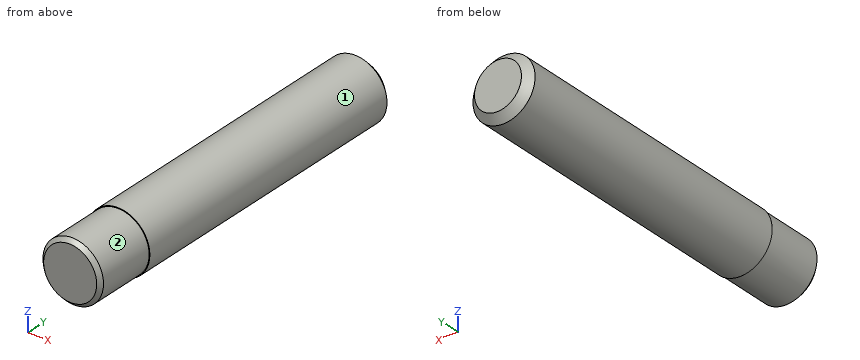
Solid Edge part; units mm, degrees
sketch "Sketch1" plane through (0, 0, 0) normal (0, -1, 0) x (1, 0, 0)
  circle A0 centre (0, 0) radius 4
extrude "Protrusion1" add sketch "Sketch1" along normal mid plane 48
sketch "Sketch2" plane through (0, 24, 0) normal (0, 1, 0) x (1, 0, 0)
  circle A0 centre (0, 0) radius 4.1
extrude "Ausprägung_2" add sketch "Sketch2" against normal blind 40
cosmetic_thread "Thread1"
chamfer "Fase_2" distance 1 angle 45 1 edges at (-4.1, 24, 0)
chamfer "Fase_3" distance 0.5 angle 45 1 edges at (-4, -24, 0)
The model under review builds one solid part; all positions refer to its coordinate system, in mm. Face numbers are marked on the shaded views. A direction names the side the tool comes from. Round coordinates to 2 decimals unless told otherwise and drop trailing zeros. Write each loop counter-clockwise with the first axis right and the second up, starting at its lowest first coordinate (ties: lowest second). Pieces come first, ordered by that corner, then holes. Notation, with made-up numbers: M 86,63 L 145,63 A17 ccw 145,74 Z; hole C 39,-13 d9. An arc over 180 degrees is marked long. Use a Markdown table: item, result. Add a question column.
Q1. Insertion check: pin 1 (2 mm diameter, centred on x = 2.5, y = 16, fed in from +Z); pin 2 (1.5 mm diameter, centred on x = -3, y = 18, fed in from +Z); pin 3 (1.5 mm diameter, centred on x = 1.5, y = 16, fed in from +Z). Each pin has a flat end and moves straight along its axis. Give the tip position at first contact, or say it passes through.
Q2. Machinability: for the marked faces 1 and 2, which of the approach directions +Z, -Z, +X, -X, +Y, -Y give a long, thin tool a straight path to every point of the face, cutting with its end or side? Answer none if there is none.
Q3. To check wall thickness, follow line 1 (Z direction, x = -0.25, y = 15.5); line 2 (X direction, y = -20.5, z = 0.25); line 3 (X direction, y = 0, z = -3.25). State the ranges of each line that lie inside material, in increasing order.
Q4. We need section A-A, the plane y = -13.5. State the section outline as (x, z) points, plus the area to 3 significant figures.
Findings below:
| question | item | result |
|---|---|---|
| 1 | pin 1 | stops at z = 3.82 |
| 1 | pin 2 | stops at z = 3.43 |
| 1 | pin 3 | stops at z = 4.03 |
| 2 | face 1 | +Y, -Y |
| 2 | face 2 | -Y |
| 3 | line 1 | z = -4.09 to 4.09 |
| 3 | line 2 | x = -3.99 to 3.99 |
| 3 | line 3 | x = -2.5 to 2.5 |
| 4 | outline | C 0,0 d8.2 |
| 4 | area | 52.8 mm² |
